The drawing under review shows one solid part. Ordinate dimensions are in mm from its lowest x, y, z. A direction names the side the tool comes from. Give positions to 0.01 mm unless a question says otherwise; leave off trailing zeros. Loops run counter-clockwise (first coordinate to the right, second up) from the corner with the lowest first, then second, coordinate; pieces in that order, holes last.
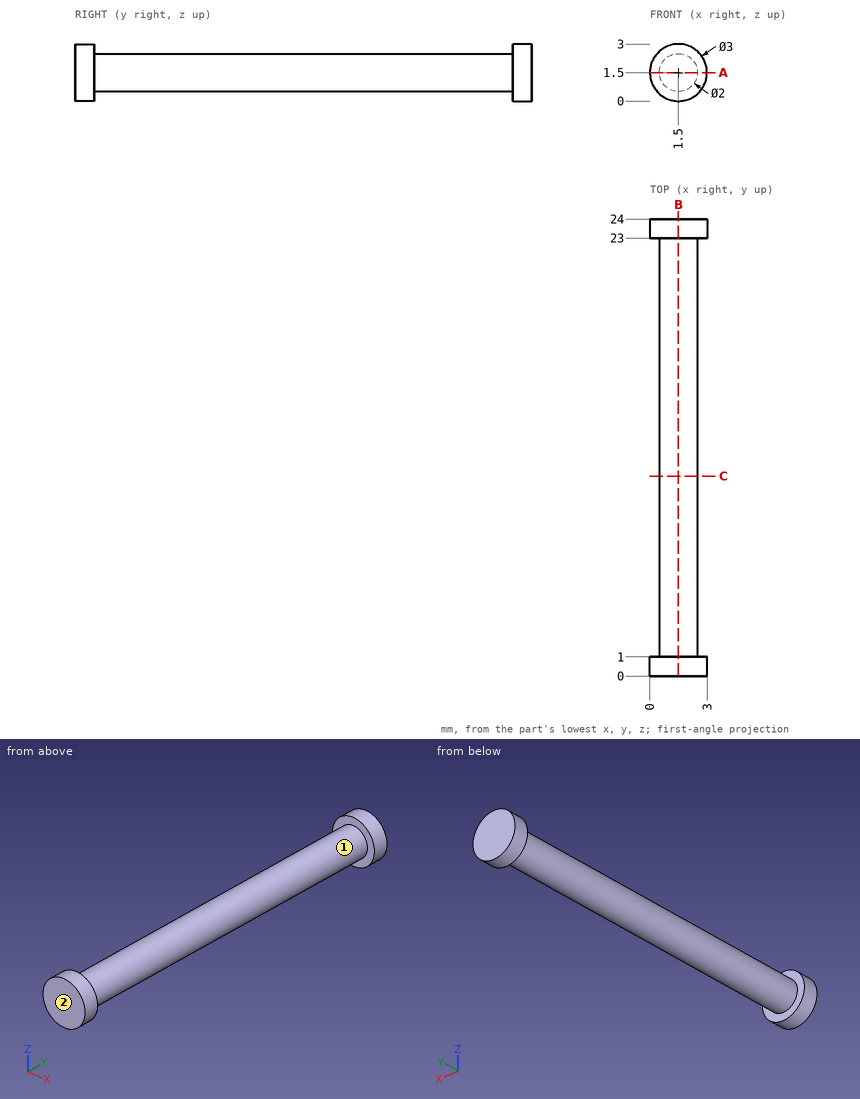
Item 1: Tool access review of the marked faces 1 and 2: name each direction out of +Z, -Z, +X, -X, +Y, -Y from which nothing blocks a thin tool from reaching the whole face with its end or side.
Answer:
face 1: none
face 2: +Z, -Z, +X, -X, -Y
Item 2: Take a section at A-A on z = 1.5. Give the boundary of the cut face in (x, y), and give its area (3 significant figures).
Answer:
outline: (0, 0) - (3, 0) - (3, 1) - (2.5, 1) - (2.5, 23) - (3, 23) - (3, 24) - (0, 24) - (0, 23) - (0.5, 23) - (0.5, 1) - (0, 1) - close
area: 50.0 mm2
Item 3: Take a section at B-B on x = 1.5. Give the boundary of the cut face in (y, z), and give its area (3 significant figures).
Answer:
outline: (0, 0) - (1, 0) - (1, 0.5) - (23, 0.5) - (23, 0) - (24, 0) - (24, 3) - (23, 3) - (23, 2.5) - (1, 2.5) - (1, 3) - (0, 3) - close
area: 50.0 mm2
Item 4: Take a section at C-C on y = 10.5. Give the boundary of the cut face in (x, z).
Answer:
outline: circle Ø2 at (1.5, 1.5)
Item 5: Clearance check with flat-ended pins moving along their axes: pin 1 Ø1.5 at (y, z) = (18.5, 2) entering from +X; pin 2 Ø1.5 at (x, y) = (2, 5.5) entering from -Z. State where each tip first meets the part, or that it passes through.
Answer:
pin 1: stops at x = 2.5
pin 2: stops at z = 0.5
Item 6: For L1, parallel to Y at x = 1.6, z = 0.2; L2, parallel to Z at x = 1.55, y = 18; L3, parallel to Z at x = 0.7, y = 18.5, list the stretches that pass through material, from the lowest coordinate up.
Answer:
L1: y = 0 to 1, 23 to 24
L2: z = 0.5 to 2.5
L3: z = 0.9 to 2.1
